```python
from build123d import *

# Parameters (mm, degrees)
EXTRUDE_1_DEPTH           = 20
SKETCH_4_R                = 13.999999999999998
EXTRUDE_2_DEPTH           = 5
HOLE_WIZARD_1_D           = 13.5
HOLE_WIZARD_1_DEPTH       = 57
HOLE_WIZARD_1_CBORE_D     = 20
HOLE_WIZARD_1_CBORE_DEPTH = 18
HOLE_WIZARD_1_TIP         = 4.055809178436032
CHAMFER_2_SIZE            = 20
CUT_EXTRUDE_1_DEPTH       = 5
SKETCH_10_R               = 5.000000000000005
CUT_EXTRUDE_2_DEPTH       = 5
CUT_EXTRUDE_3_DEPTH       = 148.73117477364084
CHAMFER_1_SIZE            = 2
SKETCH_12_W               = 150
SKETCH_12_H               = 89.99999999999999
CUT_EXTRUDE_4_DEPTH       = 148.1376906166466
FILLET_1_R                = 10
CHAMFER_3_SIZE            = 1
HOLE_WIZARD_M5_1_D        = 4.2
HOLE_WIZARD_M5_1_DEPTH    = 12.4
HOLE_WIZARD_M5_1_TIP      = 1.2618072999578767
HOLE_WIZARD_M5_2_D        = 4.2
HOLE_WIZARD_M5_2_DEPTH    = 12.4
HOLE_WIZARD_M5_2_TIP      = 1.2618072999578767


with BuildPart() as part:
    # 草图1 → 凸台-拉伸1 (new body)
    with BuildSketch(Plane.XY):
        Polygon((-103.49999999999999, 103.50000000000003), (103.50000000000001, 103.50000000000003), (103.50000000000001, -103.49999999999999), (-103.49999999999996, -103.49999999999999), align=None)
    extrude(amount=EXTRUDE_1_DEPTH)

    # 草图4 → 凸台-拉伸2 (add)
    with BuildSketch(Plane.XY.offset(20)):
        with Locations((-78.5, -78.5)):
            Circle(SKETCH_4_R)
        with Locations((-78.5, 78.5)):
            Circle(SKETCH_4_R)
        with Locations((78.5, 78.5)):
            Circle(SKETCH_4_R)
        with Locations((78.5, -78.5)):
            Circle(SKETCH_4_R)
    extrude(amount=EXTRUDE_2_DEPTH)

    # 打孔尺寸(%根据)内六角圆柱头螺钉的类型1
    with Locations(Plane.XY.offset(25)):
        with Locations((-78.5, -78.5), (-78.5, 78.5), (78.5, 78.5), (78.5, -78.5)):
            CounterBoreHole(HOLE_WIZARD_1_D / 2, HOLE_WIZARD_1_CBORE_D / 2, HOLE_WIZARD_1_CBORE_DEPTH, depth=HOLE_WIZARD_1_DEPTH)
            with Locations((0, 0, -(HOLE_WIZARD_1_DEPTH + HOLE_WIZARD_1_TIP / 2))):  # 118° drill point
                Cone(0, HOLE_WIZARD_1_D / 2, HOLE_WIZARD_1_TIP, mode=Mode.SUBTRACT)

    # 倒角2
    chamfer_2_edges = [part.edges().sort_by_distance(p)[0] for p in [
        (103.50000000000001, -103.49999999999999, 10),
        (-103.49999999999996, -103.49999999999999, 10),
        (-103.49999999999999, 103.50000000000003, 10),
        (103.50000000000001, 103.50000000000003, 10),
    ]]
    chamfer(chamfer_2_edges, length=CHAMFER_2_SIZE)

    # 草图9 → 切除-拉伸1 (cut)
    with BuildSketch(Plane.XY.offset(20)):
        Polygon((90, 60.000000000000014), (-90, 59.999999999999986), (-89.99999999999999, -60), (90.00000000000001, -59.999999999999986), align=None)
    extrude(amount=-CUT_EXTRUDE_1_DEPTH, mode=Mode.SUBTRACT)

    # 草图10 → 切除-拉伸2 (cut)
    with BuildSketch(Plane.XY.offset(20)):
        with Locations((90.00000000000001, -59.999999999999986)):
            Circle(SKETCH_10_R)
        with Locations((-89.99999999999999, -60)):
            Circle(SKETCH_10_R)
        with Locations((90, 60.000000000000014)):
            Circle(SKETCH_10_R)
        with Locations((-90, 59.999999999999986)):
            Circle(SKETCH_10_R)
    extrude(amount=-CUT_EXTRUDE_2_DEPTH, mode=Mode.SUBTRACT)

    # 草图11 → 切除-拉伸3 (cut, through all)
    with BuildSketch(Plane.XY.offset(20)):
        with BuildLine():
            Line((45.000000000000036, -92.49999999999997), (-44.99999999999998, -92.5))
            ThreePointArc((-44.99999999999998, -92.5), (-57.499999999999964, -80.00000000000001), (-44.99999999999998, -67.50000000000003))
            Line((-44.99999999999998, -67.50000000000003), (45.00000000000001, -67.5))
            ThreePointArc((45.00000000000001, -67.5), (57.50000000000001, -79.99999999999997), (45.000000000000036, -92.49999999999997))
        make_face()
        with BuildLine():
            Line((45.000000000000014, 67.50000000000004), (-45, 67.50000000000001))
            ThreePointArc((-45, 67.50000000000001), (-57.500000000000014, 80.00000000000001), (-45, 92.50000000000003))
            Line((-45, 92.50000000000003), (44.999999999999986, 92.50000000000006))
            ThreePointArc((44.999999999999986, 92.50000000000006), (57.5, 80.00000000000006), (45.000000000000014, 67.50000000000004))
        make_face()
    extrude(amount=-CUT_EXTRUDE_3_DEPTH, mode=Mode.SUBTRACT)

    # 倒角1
    chamfer_1_edges = [part.edges().sort_by_distance(p)[0] for p in [
        (57.50000000000001, -79.99999999999997, 0),
        (2.487e-14, -92.49999999999999, 0),
        (-57.49999999999997, -80.00000000000001, 0),
        (1.066e-14, -67.50000000000003, 0),
        (57.50000000000001, -79.99999999999997, 20),
        (1.421e-14, -67.50000000000001, 20),
        (-57.49999999999997, -80.00000000000001, 20),
        (2.842e-14, -92.49999999999999, 20),
        (57.50000000000001, 80.00000000000007, 0),
        (7.11e-15, 67.50000000000003, 0),
        (-57.50000000000001, 80.00000000000003, 0),
        (-1.066e-14, 92.50000000000003, 0),
        (57.50000000000001, 80.00000000000007, 20),
        (-7.11e-15, 92.50000000000004, 20),
        (-57.50000000000001, 80.00000000000003, 20),
        (7.11e-15, 67.50000000000003, 20),
        (1.421e-14, 103.50000000000003, 0),
        (1.421e-14, 103.50000000000003, 20),
        (103.50000000000001, 2.842e-14, 0),
        (2.842e-14, -103.49999999999999, 0),
        (-103.49999999999997, 1.421e-14, 0),
        (93.50000000000001, -93.49999999999999, 0),
        (-93.49999999999996, -93.5, 0),
        (-93.49999999999999, 93.50000000000003, 0),
        (93.50000000000001, 93.50000000000004, 0),
        (103.50000000000001, 2.842e-14, 20),
        (-103.49999999999997, 1.421e-14, 20),
        (2.842e-14, -103.49999999999999, 20),
        (93.50000000000001, -93.49999999999999, 20),
        (-93.49999999999996, -93.5, 20),
        (-93.49999999999999, 93.50000000000003, 20),
        (93.50000000000001, 93.50000000000004, 20),
    ]]
    chamfer(chamfer_1_edges, length=CHAMFER_1_SIZE)

    # 草图12 → 切除-拉伸4 (cut, through all)
    with BuildSketch(Plane.XY.offset(15)):
        Rectangle(SKETCH_12_W, SKETCH_12_H)
    extrude(amount=-CUT_EXTRUDE_4_DEPTH, mode=Mode.SUBTRACT)

    # 圆角1
    fillet_1_edges = [part.edges().sort_by_distance(p)[0] for p in [
        (-75, -45, 7.5),
        (-75, 44.999999999999986, 7.5),
        (74.99999999999999, 44.999999999999986, 7.5),
        (74.99999999999999, -45, 7.5),
    ]]
    fillet(fillet_1_edges, radius=FILLET_1_R)

    # 倒角3
    chamfer_3_edges = [part.edges().sort_by_distance(p)[0] for p in [
        (1.421e-14, -59.99999999999999, 20),
        (90, 2.132e-14, 20),
        (0, 60, 20),
        (-90, -7.11e-15, 20),
        (-1.421e-14, 44.999999999999986, 15),
        (-7.11e-15, 44.999999999999986, 0),
        (74.99999999999999, -7.11e-15, 15),
        (74.99999999999999, -7.11e-15, 0),
        (-75, -7.11e-15, 15),
        (-75, -7.11e-15, 0),
        (-1.421e-14, -45, 15),
        (0, -45, 0),
        (72.07106781186546, 42.07106781186546, 15),
        (72.07106781186546, 42.071067811865454, 0),
        (-72.07106781186548, 42.07106781186546, 15),
        (-72.07106781186548, 42.07106781186546, 0),
        (-72.07106781186548, -42.071067811865476, 15),
        (-72.07106781186548, -42.071067811865476, 0),
        (72.07106781186548, -42.071067811865476, 15),
        (72.07106781186548, -42.071067811865476, 0),
    ]]
    chamfer(chamfer_3_edges, length=CHAMFER_3_SIZE)

    # M5 螺纹孔1
    with Locations(Plane.XY.offset(15)):
        with Locations((77.5, -53), (-77.5, -53), (-82.5, 52), (82.5, 52)):
            Hole(HOLE_WIZARD_M5_1_D / 2, depth=HOLE_WIZARD_M5_1_DEPTH)
            with Locations((0, 0, -(HOLE_WIZARD_M5_1_DEPTH + HOLE_WIZARD_M5_1_TIP / 2))):  # 118° drill point
                Cone(0, HOLE_WIZARD_M5_1_D / 2, HOLE_WIZARD_M5_1_TIP, mode=Mode.SUBTRACT)

    # M5 螺纹孔2
    with Locations(Plane(origin=(0, 103.50000000000003, 0), x_dir=(1, 0, 0), z_dir=(0, 1, 0))):
        with Locations((-65, -10), (65, -10)):
            Hole(HOLE_WIZARD_M5_2_D / 2, depth=HOLE_WIZARD_M5_2_DEPTH)
            with Locations((0, 0, -(HOLE_WIZARD_M5_2_DEPTH + HOLE_WIZARD_M5_2_TIP / 2))):  # 118° drill point
                Cone(0, HOLE_WIZARD_M5_2_D / 2, HOLE_WIZARD_M5_2_TIP, mode=Mode.SUBTRACT)


solid = part.part
```
CAD build for the part. Positions are in the model's coordinates, mm. A direction names the side the tool comes from. Coordinates: 2 decimals unless noted, no trailing zeros. Write each loop counter-clockwise with the first axis right and the second up, starting at its lowest first coordinate (ties: lowest second). Pieces come first, ordered by that corner, then holes.
(1) Flat gauge pins, fed straight in: pin 1 (6 mm diameter, centred on x = -90, y = 60, fed in from +Z); pin 2 (23 mm diameter, centred on x = 78.5, y = 78.5, fed in from -Z); pin 3 (12 mm diameter, centred on x = -36, y = 68, fed in from +Z). Where does each tip first touch, or does it go through?
(2) Cut at A-A, the plane y = 31.5. List the corners of the cut face in (x, z), and give its area (3 significant figures).
(3) Cut at B-B, the plane x = 22. Count the separate pieces of the cut face and the enclosed holes in it, and give its area (3 significant figures).
(4) Two-plate mould, pull along Y, no slides. Class faces 1 (the face through (103.5, 1, 10)), 2 (the face through (-93, 64, 18)): +Y half, -Y half, draft (parallel to the pull), parting line (faces both ways), or undercut.
(5) Drill centre lines: probe 1 along Y at (x, z) = (-34.5, 12.5); probe 2 along X at (y, z) = (-53, 8.5); probe 3 along X at (y, z) = (52, 11.5). Where is each one in solid material? Low to high.
(6) 3-axis set-ups, long thin cutter, end or side, ignore diameter. For faces 3 (the face through (-75, 0, 8)), 4 (the face through (57.816, -80.282, 1.681)), 5 (the face through (-72.27, 42.11, 14.17)), 6 (the face through (-72, 69, 25)): which of +Z, -Z, +X, -X, +Y, -Y reach the whole face in a straight line?
Geometry says:
1. pin 1: stops at z = 15
1. pin 2: stops at z = 0
1. pin 3: stops at z = 20
2. outline: (-103.5, 2) - (-101.5, 0) - (-76, 0) - (-75, 1) - (-75, 14) - (-76, 15) - (-90, 15) - (-90, 19) - (-91, 20) - (-101.5, 20) - (-103.5, 18) - close; (75, 1) - (76, 0) - (101.5, 0) - (103.5, 2) - (103.5, 18) - (101.5, 20) - (91, 20) - (90, 19) - (90, 15) - (76, 15) - (75, 14) - close
2. area: 979 mm2
3. separate pieces: 4
3. enclosed holes: 0
3. area: 1,160 mm2
4. face 1: draft
4. face 2: undercut
5. probe 1: y = -103.5 to -92.5, -67.5 to -45, 45 to 67.5, 92.5 to 103.5
5. probe 2: x = -103.5 to -79.6, -75.4 to 75.4, 79.6 to 103.5
5. probe 3: x = -103.5 to -84.6, -80.4 to 80.4, 84.6 to 103.5
6. face 3: +Z, -Z
6. face 4: -Z
6. face 5: +Z
6. face 6: +Z, +X, -X, +Y, -Y
